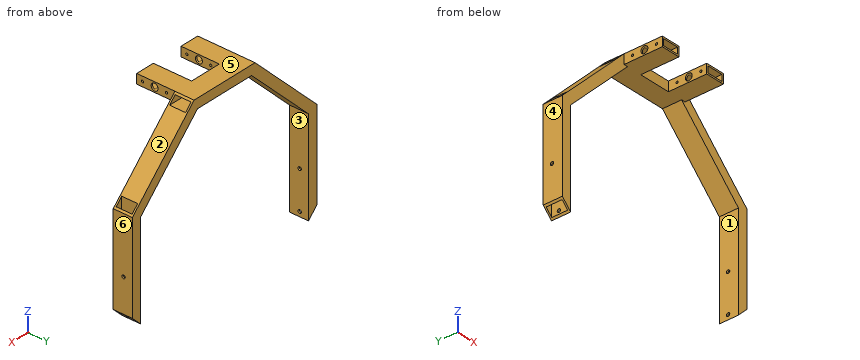
Autodesk Inventor part; units mm, degrees
ref_plane "Work Plane1" through (0, 0, -330.2) normal (0, 0, 1) x (1, 0, 0)
ref_plane "Work Plane2" through (-192.0875, -19.05, -9.525) normal (0, 0, 1) x (1, 0, 0)
ref_plane "Work Plane4" through (0, 19.05, -139.7) normal (-1, 0, 0) x (0, 0, -1)
sketch "Sketch1" plane through (0, 0, 0) normal (0, 1, 0) x (-1, 0, 0)
  line L0 (0, 0) -> (201.6125, 0)
  line L1 (201.6125, 0) -> (201.6125, -330.2)
  line L2 (0, 0) -> (0, -330.2) construction
  line L3 (0, 0) -> (-201.6125, 0)
  line L4 (-201.6125, 0) -> (-201.6125, -330.2)
  dimension "d0" = 201.6125
  dimension "d1" = 330.2
  dimension "d2" = 330.2
ref_plane "Work Plane1" through (0, 0, -330.2) normal (0, 0, 1) x (1, 0, 0)
sketch "Sketch3" plane through (0, 0, -330.2) normal (0, 0, 1) x (1, 0, 0)
  line L0 (211.1375, -19.05) -> (192.0875, -19.05)
  line L1 (192.0875, -19.05) -> (192.0875, 19.05)
  line L2 (192.0875, 19.05) -> (211.1375, 19.05)
  line L3 (211.1375, 19.05) -> (211.1375, -19.05)
  line L4 (211.1375, -19.05) -> (192.0875, 19.05) construction
  line L5 (192.0875, -19.05) -> (211.1375, 19.05) construction
  line L6 (207.9625, -15.875) -> (195.2625, -15.875)
  line L7 (195.2625, -15.875) -> (195.2625, 15.875)
  line L8 (195.2625, 15.875) -> (207.9625, 15.875)
  line L9 (207.9625, 15.875) -> (207.9625, -15.875)
  line L10 (207.9625, -15.875) -> (195.2625, 15.875) construction
  line L11 (195.2625, -15.875) -> (207.9625, 15.875) construction
  point P0 (0, 0)
  point P1 (201.6125, 0)
  dimension "d4" = 38.1
  dimension "d5" = 19.05
  dimension "d6" = 201.6125
  dimension "d7" = 3.175
  dimension "d8" = 3.175
sweep "Sweep1" add profiles "Sketch3" path "Sketch1"
ref_plane "Work Plane2" through (-192.0875, -19.05, -9.525) normal (0, 0, 1) x (1, 0, 0)
sketch "Sketch12" plane through (-211.1375, 19.05, 9.525) normal (0, 1, 0) x (1, 0, 0)
  line L0 (406.4, 15.875) -> (15.875, 15.875)
  line L1 (19.05, 19.05) -> (19.05, 339.725)
  line L2 (19.05, 149.225) -> (149.225, 19.05)
  line L3 (403.225, 19.05) -> (19.05, 19.05)
  line L4 (19.05, 122.2842) -> (122.2842, 19.05)
  line L5 (19.05, 149.225) -> (19.05, 122.2842)
  line L6 (122.2842, 19.05) -> (149.225, 19.05)
  line L7 (211.1375, 9.525) -> (211.1375, 339.725) construction
  line L8 (403.225, 19.05) -> (403.225, 339.725)
  line L9 (403.225, 149.225) -> (273.05, 19.05)
  line L10 (19.05, 19.05) -> (403.225, 19.05)
  line L11 (403.225, 122.2842) -> (299.9908, 19.05)
  dimension "d50" = 130.175
  dimension "d51" = 130.175
  dimension "d52" = 19.05
  dimension "d55" = 330.2
extrude "Extrusion5" add sketch "Sketch12" against normal blind 38.1 contours L9 L8 L11 L3 | L1 L2 L3 L4
sketch "Sketch14" plane through (-211.1375, 19.05, 9.525) normal (0, 1, 0) x (1, 0, 0)
  line L0 (0, 0) -> (0, 339.725)
  line L1 (0, 141.3342) -> (141.3342, 0)
  line L2 (422.275, 0) -> (0, 0)
  line L3 (19.05, 122.2842) -> (122.2842, 19.05)
  line L4 (0, 141.3342) -> (0, 0)
  line L5 (211.1375, 9.525) -> (211.1375, 339.725) construction
  dimension "d58" = 330.2
extrude "Extrusion6" cut sketch "Sketch14" against normal blind 38.1
sketch "Sketch15" plane through (211.1375, 19.05, 9.525) normal (0, 1, 0) x (1, 0, 0)
  line L0 (0, 0) -> (-280.9408, 0)
  line L1 (-141.3342, 0) -> (0, 141.3342)
  line L2 (0, 339.725) -> (0, 0)
  line L3 (-122.2842, 19.05) -> (-19.05, 122.2842)
  line L4 (-141.3342, 0) -> (0, 0)
  point P0 (-211.1375, 9.525)
extrude "Extrusion7" cut sketch "Sketch15" against normal blind 38.1
sketch "Sketch17" plane through (192.0875, 19.05, -330.2) normal (0, 1, 0) x (1, 0, 0)
  line L0 (-384.175, -190.5) -> (-384.175, 0)
  line L1 (-384.175, 0) -> (-403.225, -19.05)
  line L2 (-403.225, -198.3908) -> (-403.225, 0)
  line L3 (-403.225, -19.05) -> (-403.225, 0)
  line L4 (-403.225, 0) -> (-384.175, 0)
  point P0 (-192.0875, -330.2)
  dimension "d63" = 45
extrude "Extrusion8" cut sketch "Sketch17" against normal through all
sketch "Sketch18" plane through (192.0875, 19.05, -330.2) normal (0, 1, 0) x (1, 0, 0)
  line L0 (0, 0) -> (0, -190.5)
  line L1 (0, 0) -> (19.05, -19.05)
  line L2 (19.05, 0) -> (19.05, -198.3908)
  line L3 (19.05, -19.05) -> (19.05, 0)
  line L4 (19.05, 0) -> (0, 0)
  line L5 (19.05, 0) -> (0, 0)
  point P0 (-192.0875, -330.2)
  dimension "d66" = 45
extrude "Extrusion9" cut sketch "Sketch18" against normal through all
sketch "Sketch19" plane through (-69.8033, -19.05, 9.525) normal (0, -1, 0) x (1, 0, 0)
  line L0 (139.6065, 0) -> (0, 0)
  line L1 (131.7158, -19.05) -> (7.8908, -19.05)
  line L2 (0, 0) -> (38.1, 0)
  line L3 (38.1, 0) -> (38.1, -19.05)
  line L4 (38.1, -19.05) -> (0, -19.05)
  line L5 (0, -19.05) -> (0, 0)
  line L6 (280.9408, -141.3342) -> (139.6065, 0)
  line L7 (139.6065, 0) -> (101.5065, 0)
  line L8 (101.5065, 0) -> (101.5065, -19.05)
  line L9 (101.5065, -19.05) -> (139.6065, -19.05)
  line L10 (139.6065, -19.05) -> (139.6065, 0)
  line L11 (0, -9.525) -> (139.6065, -9.525) construction
  line L12 (120.5565, 0) -> (120.5565, -19.05) construction
  line L13 (19.05, 0) -> (19.05, -19.05) construction
  line L14 (131.7158, -19.05) -> (7.8908, -19.05) construction
  line L15 (3.175, -15.875) -> (34.925, -15.875)
  line L16 (34.925, -15.875) -> (34.925, -3.175)
  line L17 (34.925, -3.175) -> (3.175, -3.175)
  line L18 (3.175, -3.175) -> (3.175, -15.875)
  line L19 (3.175, -15.875) -> (34.925, -3.175) construction
  line L20 (34.925, -15.875) -> (3.175, -3.175) construction
  line L21 (104.6815, -15.875) -> (136.4315, -15.875)
  line L22 (136.4315, -15.875) -> (136.4315, -3.175)
  line L23 (136.4315, -3.175) -> (104.6815, -3.175)
  line L24 (104.6815, -3.175) -> (104.6815, -15.875)
  line L25 (104.6815, -15.875) -> (136.4315, -3.175) construction
  line L26 (136.4315, -15.875) -> (104.6815, -3.175) construction
  point P0 (69.8033, -9.525)
  point P1 (19.05, -9.525)
  point P2 (120.5565, -9.525)
  dimension "d69" = 38.1
  dimension "d70" = 38.1
  dimension "d71" = 3.175
  dimension "d72" = 3.175
  dimension "d73" = 3.175
  dimension "d74" = 3.175
extrude "Extrusion10" add sketch "Sketch19" along normal blind 76.2 contours L10 L9 L1 L8 L0 | L3 L1 L4 L5 L0
sketch "Sketch20" plane through (69.8033, -19.05, 9.525) normal (1, 0, 0) x (0, 0, -1)
  circle A0 centre (9.525, -40.5384) radius 6.8707
  line L0 (141.3342, 0) -> (0, 0)
  point P0 (9.525, 19.05)
  dimension "d77" = 13.7414
  dimension "d78" = 40.5384
extrude "Extrusion11" cut sketch "Sketch20" against normal through all
ref_plane "Work Plane4" through (0, 19.05, -139.7) normal (-1, 0, 0) x (0, 0, -1)
ref_plane "Work Plane3" through (-192.0875, 19.05, -139.7) normal (-1, 0, 0) x (0, 0, -1)
sketch "Sketch21" plane through (-211.1375, -19.05, -131.8092) normal (-1, 0, 0) x (0, 0, 1)
  line L0 (-179.3408, 38.1) -> (-179.3408, 0)
  line L1 (0, 0) -> (-179.3408, 0)
  line L2 (0, 0) -> (0, 38.1)
  line L3 (0, 38.1) -> (-179.3408, 38.1)
  circle A0 centre (-112.6658, 20.6375) radius 3.3735
  circle A1 centre (-188.8658, 20.6375) radius 3.3735
  point P0 (131.8092, 19.05)
extrude "Extrusion12" cut sketch "Sketch21" against normal through all contours A0 | A1
sketch "Sketch22" plane through (69.8033, -19.05, 9.525) normal (1, 0, 0) x (0, 0, -1)
  circle A0 centre (9.525, -40.8462) radius 23.8125 construction
  arc A1 (15.875, -37.9147) -> (3.175, -37.9147) centre (9.525, -40.5384) ccw construction
  line L0 (9.525, -40.5384) -> (9.525, -17.0337) construction
  line L1 (9.525, -40.5384) -> (9.525, -64.6587) construction
  point P0 (9.525, 19.05)
  point P1 (-29.4266, 19.05)
  dimension "d84" = 47.625
hole "Hole3" at (69.8033, 0, 38.9516) at (69.8033, -36.0837, 0) at (69.8033, -83.7087, 0) direction (-1, 0, 0) diameter 4.4958 end through all
equation "\"d0\" = 0.5 * width"
equation "\"d1\" = length"
equation "\"d2\" = length"
equation "\"d4\" = tubingLength"
equation "\"d5\" = tubingWidth"
equation "\"d7\" = tubeingWallWidth"
equation "\"d8\" = tubeingWallWidth"
equation "\"d55\" = length"
equation "\"d58\" = length"
equation "\"d77\" = diamForAxel"
equation "\"width\" = 403.225"
equation "\"length\" = 330.2"
equation "\"tubingWidth\" = 19.05"
equation "\"tubingLength\" = 38.1"
equation "\"tubeingWallWidth\" = 3.175"
equation "\"d3\" = -length"
equation "\"diamForAxel\" = 13.7414"
properties part number "ShooterFrameV02" material "Aluminum 6061"
Read the model definition and answer for the solid it produces. Units are mm, in the model's axes. Face numbers are marked on the shaded views. A direction names the side the tool comes from. Give positions to 0.01 mm unless a question says otherwise; leave off trailing zeros. Loops run counter-clockwise (first coordinate to the right, second up) from the corner with the lowest first, then second, coordinate; pieces in that order, holes last. Notation, with made-up numbers: (30.5, 63.25) -> (80.5, 63.25) arc R32 cw to (80.5, 98.25) -> close; hole circle Ø6 at (-5.75, 75). An arc over 180 degrees is marked (long way). Use a Markdown table: item, result.
Q1. A tool of negligible diameter and unlimited length cuts with its end or side. For the marked faces 1 and 2, from which of +Z, -Z, +X, -X, +Y, -Y can it reach the whole face along a straight path? Write none if from no direction.
Solved:
| item | result |
|---|---|
| face 1 | -Z, +Y, -Y |
| face 2 | +Z, +X, +Y, -Y |
Q2. Each of these flat-tipped pins is pushed along its axis until it touches: pin 1 (6.5 mm diameter, centred on y = -86.5, z = -2, fed in from -X); pin 2 (6 mm diameter, centred on y = -36.08, z = 0, fed in from +X); pin 3 (9.5 mm diameter, centred on x = -46.5, y = -34.5, fed in from -Z) (3 decimals); pin 4 (4 mm diameter, centred on y = -83.71, z = 0, fed in from +X). Where does it stop, or does it pass through?
Solved:
| item | result |
|---|---|
| pin 1 | stops at x = -69.8 |
| pin 2 | stops at x = 69.8 |
| pin 3 | stops at z = -9.525 |
| pin 4 | passes through |
Q3. Section B-B, the plane y = -24 is taken. Determine the outline of the cut face in (x, z) (3 decimals).
Solved:
| item | result |
|---|---|
| outline | (-69.803, -9.525) -> (-31.703, -9.525) -> (-31.703, 9.525) -> (-69.803, 9.525) -> close; (31.703, -9.525) -> (69.803, -9.525) -> (69.803, 9.525) -> (31.703, 9.525) -> close; hole (-66.628, -6.35) -> (-34.878, -6.35) -> (-34.878, 6.35) -> (-66.628, 6.35) -> close; hole (34.878, -6.35) -> (66.628, -6.35) -> (66.628, 6.35) -> (34.878, 6.35) -> close |
Q4. Determine the mould class of the marked faces 3, 4, 5 and 6 for opening direction X: pulls with the +X half, pulls with the -X half, needs draft (parallel to the pull), parting line crosses it, or undercut.
Solved:
| item | result |
|---|---|
| face 3 | undercut |
| face 4 | pulls with the -X half |
| face 5 | needs draft |
| face 6 | pulls with the +X half |
Q5. Section C-C, the plane z = -73.5 is taken. Determine the outline of the cut face in (x, y).
Solved:
| item | result |
|---|---|
| outline | (-152.83, -19.05) -> (-125.89, -19.05) -> (-125.89, 19.05) -> (-152.83, 19.05) -> close; (125.89, -19.05) -> (152.83, -19.05) -> (152.83, 19.05) -> (125.89, 19.05) -> close |
Q6. Section A-A, the plane z = -273 is taken. Count the separate pieces of the cut face and the enclosed holes in it, then the cut area to 3 significant figures.
Solved:
| item | result |
|---|---|
| separate pieces | 2 |
| enclosed holes | 2 |
| area | 645 mm^2 |
Q7. Section D-D, the plane x = -93 is taken. Determine the outline of the cut face in (y, z).
Solved:
| item | result |
|---|---|
| outline | (-19.05, -40.61) -> (19.05, -40.61) -> (19.05, -13.67) -> (-19.05, -13.67) -> close |
Q8. Find the intervals of material crossed by line 1 along Y through (x, z) = (-68.1, 0) (3 decimals); line 2 along X through (y, z) = (-88.5, -5.5); line 3 along X through (y, z) = (0.5, -138.5), in increasing order.
Solved:
| item | result |
|---|---|
| line 1 | y = -95.25 to -85.957, -81.461 to -66.459, -52.718 to -38.332, -33.836 to -15.875, 15.875 to 19.05 |
| line 2 | x = -69.8 to -66.63, -34.88 to -31.7, 31.7 to 34.88, 66.63 to 69.8 |
| line 3 | x = -211.14 to -207.96, -195.26 to -190.89, 190.89 to 195.26, 207.96 to 211.14 |
